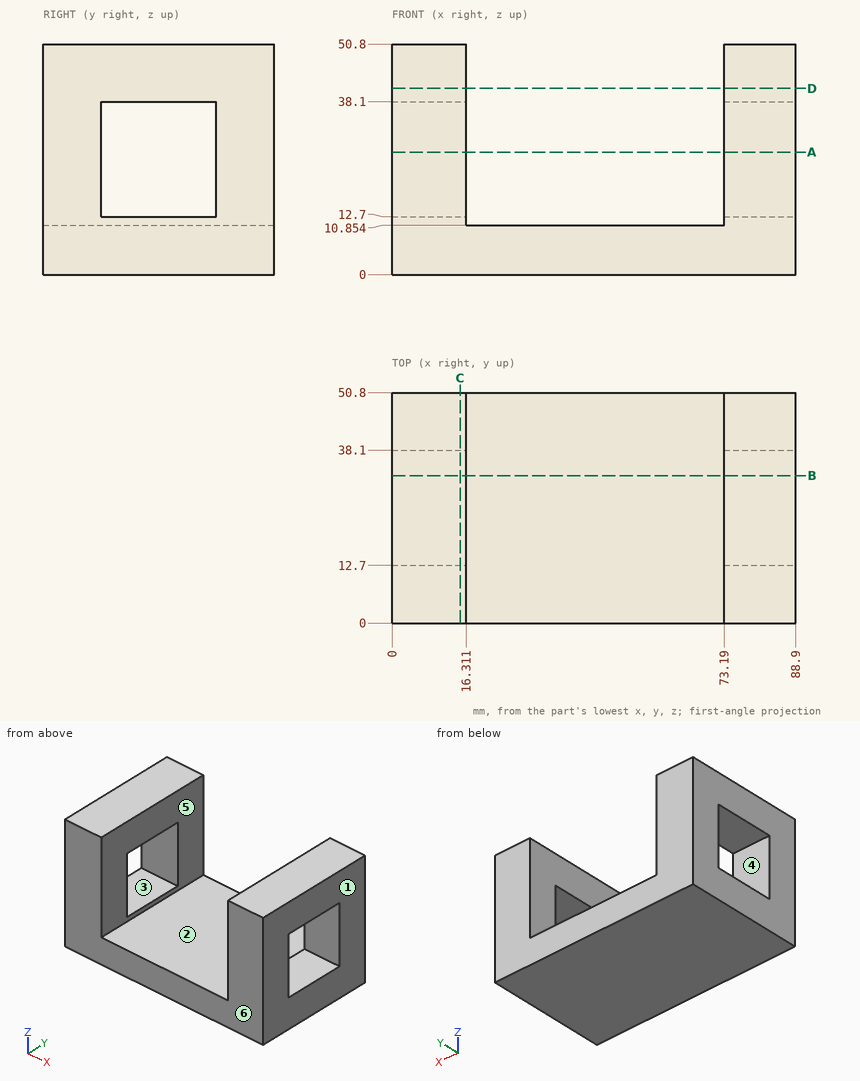
Geometry check sheet. Reference: drawing and pictorial views, mm from the part's lowest x, y, z. A direction names the side the tool comes from. Round coordinates to 2 decimals unless told otherwise and drop trailing zeros. Order: outer loops, then holes, each group sorted by start corner. A loop starts at its lowest first (then second) coordinate and runs counter-clockwise, first axis right, second up. Notation, with made-up numbers: M 44,15 L 68,15 A22 ccw 68,26 Z; hole C 51,56.5 d9. An arc over 180 degrees is marked long. Answer in a Markdown table with one row per item.
(1) Sectioned sample at B-B, the plane y = 32.5. Record the cut outline in (x, z) (1 decimal).
Responses:
| item | result |
|---|---|
| outline | M 0,0 L 88.9,0 L 88.9,12.7 L 73.2,12.7 L 73.2,10.9 L 16.3,10.9 L 16.3,12.7 L 0,12.7 Z; M 0,38.1 L 16.3,38.1 L 16.3,50.8 L 0,50.8 Z; M 73.2,38.1 L 88.9,38.1 L 88.9,50.8 L 73.2,50.8 Z |
(2) Sectioned sample at A-A, the plane z = 27. Record the cut outline in (x, y).
Responses:
| item | result |
|---|---|
| outline | M 0,0 L 16.31,0 L 16.31,12.7 L 0,12.7 Z; M 0,38.1 L 16.31,38.1 L 16.31,50.8 L 0,50.8 Z; M 73.19,0 L 88.9,0 L 88.9,12.7 L 73.19,12.7 Z; M 73.19,38.1 L 88.9,38.1 L 88.9,50.8 L 73.19,50.8 Z |
(3) Scan lines: probe 1 along X at (y, z) = (40.5, 12.5); probe 2 along Y at (x, z) = (81, 34); probe 3 along Z at (x, y) = (28, 41.5) (1 decimal). Record each from-to range of solid material in increasing order. Write a range as from..to.
Responses:
| item | result |
|---|---|
| probe 1 | x = 0..16.31, 73.19..88.9 |
| probe 2 | y = 0..12.7, 38.1..50.8 |
| probe 3 | z = 0..10.9 |
(4) Sectioned sample at C-C, the plane x = 15. Record the cut outline in (y, z), and give its area (3 significant figures).
Responses:
| item | result |
|---|---|
| outline | M 0,0 L 50.8,0 L 50.8,50.8 L 0,50.8 Z; hole M 12.7,12.7 L 38.1,12.7 L 38.1,38.1 L 12.7,38.1 Z |
| area | 1,940 mm² |
(5) Sectioned sample at D-D, the plane z = 41. Record the cut outline in (x, y).
Responses:
| item | result |
|---|---|
| outline | M 0,0 L 16.31,0 L 16.31,50.8 L 0,50.8 Z; M 73.19,0 L 88.9,0 L 88.9,50.8 L 73.19,50.8 Z |
(6) Tool access check on the marked faces 4, 5 and 6. Record the directions out of +Z, -Z, +X, -X, +Y, -Y that give a thin tool (end or side, any length) a straight path to the whole face; none if there is none.
Responses:
| item | result |
|---|---|
| face 4 | +X, -X |
| face 5 | +Z, +Y, -Y |
| face 6 | +Z, -Z, +X, -X, -Y |
(7) Draft check along X on the marked faces 1, 2 and 3. Enter one of: released by +X, released by -X, zero draft, split by the parting line, or undercut.
Responses:
| item | result |
|---|---|
| face 1 | released by +X |
| face 2 | undercut |
| face 3 | zero draft |
(8) Go/stop test with flat-tipped pins: P1, Ø12, axis at x = 55.5, y = 14, coming from the +Z side; P2, Ø12, axis at y = 24, z = 23.5, coming from the +X side. Record where each tip stops, or that it passes through.
Responses:
| item | result |
|---|---|
| P1 | stops at z = 10.85 |
| P2 | passes through |
